Read the model definition and answer for the solid it produces. Units are mm, in the model's axes. A direction names the side the tool comes from. Give positions to 0.01 mm unless a question says otherwise; leave off trailing zeros. Loops run counter-clockwise (first coordinate to the right, second up) from the corner with the lowest first, then second, coordinate; pieces in that order, holes last. Notation, with made-up numbers: (-32.5, 19) - (-25.5, 19) arc R20 ccw to (-25.5, 31) - close; hole circle Ø8 at (-36, 77). An arc over 180 degrees is marked (long way). Put each result on its own line as item: value. Start each with the question number.
1. Given pin 1 Ø1.5 at (x, z) = (1.5, -2.5) entering from +Y; pin 2 Ø2 at (x, y) = (0.5, 3) entering from +Z, each flat-ended and moving along its own axis, determine where each tip first touches the part or whether it passes through.
2. A cutting plane is placed at D-D, the plane z = 4.75. Determine the outline of the cut face in (x, y).
3. A cutting plane is placed at C-C, the plane y = -3.25. Determine the outline of the cut face in (x, z), plus the area to 3 significant figures.
4. Consider L1, parallel to Z at x = 2.5, y = -0.25; L2, parallel to Z at x = 3.45, y = 1; L3, parallel to Y at x = 0.6, z = 0.75. Determine where each line is inside the solid, lowest interval first. Write a range as from..to.
5. For a pull along Y with two mould halves and no side action, classify faces 3 (the flat face through (4, 4, 4)), 4 (the cylindrical face through (2, 0, 6)), 5 (the cylindrical face through (3.75, -4.88, 1.08)), 6 (the cylindrical face through (2, -2, 0)) as released by +Y, released by -Y, zero draft, split by the parting line, or undercut.
6. For faces 1 (the flat face through (0, 1, 2)), 2 (the flat face through (1, 6, 2)), determine the directions among +Z, -Z, +X, -X, +Y, -Y from which every point of the face is accessible in a straight line to the end or side of a thin tool.
7. A cutting plane is placed at A-A, the plane z = 0. Determine the outline of the cut face in (x, y).
Autodesk Inventor part; units mm, degrees
ref_plane "YZ Plane" through (0, 0, 0) normal (1, 0, 0) x (0, 1, 0)
ref_plane "XZ Plane" through (0, 0, 0) normal (0, 1, 0) x (-1, 0, 0)
ref_plane "XY Plane" through (0, 0, 0) normal (0, 0, 1) x (1, 0, 0)
sketch "Эскиз1" plane through (0, 0, 0) normal (1, 0, 0) x (0, 1, 0)
  circle A0 centre (0, 0) radius 7
  dimension "d0" = 14
extrude "Выдавливание1" add sketch "Эскиз1" along normal blind 1
sketch "Эскиз2" plane through (1, 0, 0) normal (1, 0, 0) x (0, 0, -1)
  circle A0 centre (0, 0) radius 6
  dimension "d3" = 12
extrude "Выдавливание2" add sketch "Эскиз2" along normal blind 3
sketch "Эскиз3" plane through (4, 0, 0) normal (1, 0, 0) x (0, 0, -1)
  circle A0 centre (0, 0) radius 2
  dimension "d6" = 4
extrude "Выдавливание3" cut sketch "Эскиз3" against normal blind 10
sketch "Эскиз4" plane through (4, 0, 0) normal (1, 0, 0) x (0, 0, -1)
  circle A0 centre (0, 0) radius 3
  circle A1 centre (0, 0) radius 5
  dimension "d9" = 6
  dimension "d10" = 10
extrude "Выдавливание4" cut sketch "Эскиз4" against normal blind 0.5
properties part number "подшипник для катков" material "Титан"
Return value:
1. pin 1: stops at y = 6.73
1. pin 2: stops at z = 6.71
2. outline: (0, -5.14) - (1, -5.14) - (1, -3.67) - (4, -3.67) - (4, -1.56) - (3.5, -1.56) - (3.5, 1.56) - (4, 1.56) - (4, 3.67) - (1, 3.67) - (1, 5.14) - (0, 5.14) - close
3. outline: (0, -6.2) - (1, -6.2) - (1, -5.04) - (4, -5.04) - (4, -3.8) - (3.5, -3.8) - (3.5, 3.8) - (4, 3.8) - (4, 5.04) - (1, 5.04) - (1, 6.2) - (0, 6.2) - close
3. area: 38.9 mm2
4. L1: z = -5.99..-1.98, 1.98..5.99
4. L2: z = -5.92..-1.73, 1.73..5.92
4. L3: y = -6.96..-1.85, 1.85..6.96
5. face 3: zero draft
5. face 4: split by the parting line
5. face 5: undercut
5. face 6: undercut
6. face 1: +Z, -Z, -X, +Y, -Y
6. face 2: +X
7. outline: (0, -7) - (1, -7) - (1, -6) - (4, -6) - (4, -5) - (3.5, -5) - (3.5, -3) - (4, -3) - (4, -2) - (0, -2) - close; (0, 2) - (4, 2) - (4, 3) - (3.5, 3) - (3.5, 5) - (4, 5) - (4, 6) - (1, 6) - (1, 7) - (0, 7) - close
